Verification items for the finished model (mm, model axes). Face numbers are marked on the shaded views. Give positions to 0.01 mm unless a question says otherwise; leave off trailing zeros. Write each loop counter-clockwise with the first axis right and the second up, starting at its lowest first coordinate (ties: lowest second). Pieces come first, ordered by that corner, then holes. Notation, with made-up numbers: (-20, 72) -> (-2, 72) arc R22 cw to (-2, 79) -> close; hole circle Ø3 at (43.5, 89). An arc over 180 degrees is marked (long way). Use CSV: the item, a comma, the result in double quotes. Start each with the question number.
```python
from build123d import *

# Parameters (mm, degrees)
SKETCH1_R           = 25
BOSS_EXTRUDE1_DEPTH = 3.175
SKETCH2_W           = 4.5
SKETCH2_H           = 2.5
CUT_EXTRUDE1_DEPTH  = 0.5


with BuildPart() as part:
    # Sketch1 → Boss-Extrude1 (new body)
    with BuildSketch(Plane(origin=(0, 0, 0), x_dir=(1, 0, 0), z_dir=(0, 1, 0))):
        Circle(SKETCH1_R)
    extrude(amount=BOSS_EXTRUDE1_DEPTH)

    # Sketch2 → Cut-Extrude1 (cut)
    with BuildSketch(Plane(origin=(0, 3.175, 0), x_dir=(1, 0, 0), z_dir=(0, 1, 0))):
        with BuildLine():
            Line((17.25, 0.25), (17.25, -5.855662433))
            Line((17.25, -5.855662433), (18.049038106, -6.316987298))
            Line((18.049038106, -6.316987298), (18.049038106, -5.25))
            Line((18.049038106, -5.25), (18.049038106, -4.816987298))
            Line((18.049038106, -4.816987298), (18.549038106, -4.816987298))
            Line((18.549038106, -4.816987298), (18.549038106, -5.25))
            Line((18.549038106, -5.25), (18.549038106, -6.5))
            Line((18.549038106, -6.5), (21.299038106, -6.5))
            Line((21.299038106, -6.5), (21.299038106, -7))
            Line((21.299038106, -7), (18.549038106, -7))
            Line((18.549038106, -7), (18.549038106, -8.25))
            Line((18.549038106, -8.25), (18.549038106, -8.683012702))
            Line((18.549038106, -8.683012702), (18.049038106, -8.683012702))
            Line((18.049038106, -8.683012702), (18.049038106, -8.25))
            Line((18.049038106, -8.25), (18.049038106, -7.183012702))
            Line((18.049038106, -7.183012702), (15.450961894, -8.683012702))
            Line((15.450961894, -8.683012702), (15.450961894, -7))
            Line((15.450961894, -7), (12.700961894, -7))
            Line((12.700961894, -7), (12.700961894, -6.5))
            Line((12.700961894, -6.5), (15.450961894, -6.5))
            Line((15.450961894, -6.5), (15.450961894, -4.816987298))
            Line((15.450961894, -4.816987298), (16.75, -5.566987298))
            Line((16.75, -5.566987298), (16.75, -0.25))
            Line((16.75, -0.25), (0.25, -0.25))
            Line((0.25, -0.25), (0.25, -24.998749969))
            ThreePointArc((0.25, -24.998749969), (0, -25), (-0.25, -24.998749969))
            Line((-0.25, -24.998749969), (-0.25, -0.25))
            Line((-0.25, -0.25), (-2.75, -0.25))
            Line((-2.75, -0.25), (-2.75, -3.25))
            Line((-2.75, -3.25), (-8.25, -3.25))
            Line((-8.25, -3.25), (-8.25, 0.25))
            Line((-8.25, 0.25), (-5.589373118, 0.25))
            Line((-5.589373118, 0.25), (-0.853083665, 4.132571689))
            Line((-0.853083665, 4.132571689), (-0.751596944, 4.215765395))
            Line((-0.751596944, 4.215765395), (-0.625482869, 4.179488852))
            Line((-0.625482869, 4.179488852), (13.035241579, 0.25))
            Line((13.035241579, 0.25), (17.25, 0.25))
        make_face()
        Polygon((-4.800684576, 0.25), (-0.297938398, 0.25), (-0.866588339, 3.47497407), align=None, mode=Mode.SUBTRACT)
        Polygon((0.209774908, 0.25), (-0.378852437, 3.588271558), (11.226526686, 0.25), align=None, mode=Mode.SUBTRACT)
        with Locations((-5.5, -1.5)):
            Rectangle(SKETCH2_W, SKETCH2_H, mode=Mode.SUBTRACT)
    extrude(amount=-CUT_EXTRUDE1_DEPTH, mode=Mode.SUBTRACT)


solid = part.part
```
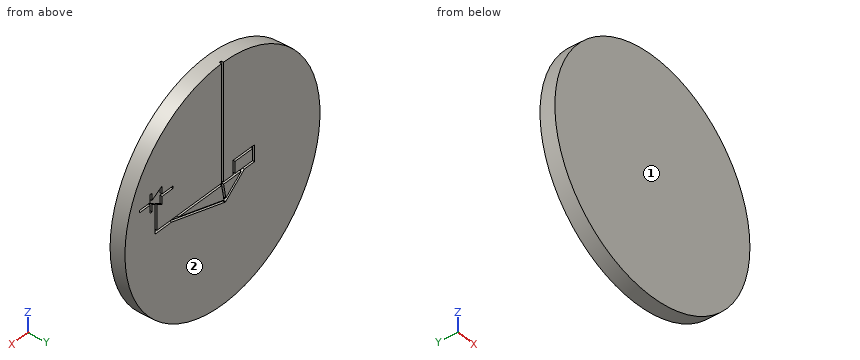
(1) Section check B-B on x = -4. Record the cut outline in (y, z) (3 decimals).
(2) Thickness scan on line 1 (Z direction, x = 16.5, y = 2.85); line 2 (Z direction, x = -0.5, y = 0.8) (3 decimals); line 3 (Z direction, x = -16.5, y = 2.7). Record the ranges inside material, lowest first. Write a range as from..to.
(3) Section check D-D on z = 11.5. Record the cut outline in (x, y) (3 decimals).
(4) Draft check along Y on the marked faces 1 and 2. Enter one of: released by +Y, released by -Y, zero draft, split by the parting line, or undercut.
(5) Section check C-C on y = 1.25. Record the cut outline in (x, z), then the cut area to 3 significant figures.
(6) Section check A-A on z = 18. Record the cut outline in (x, y) (3 decimals), then the cut area to 3 significant figures.
(7) Go/stop test with flat-tipped pins: pin 1 (0.6 mm diameter, centred on x = -5, y = 3, fed in from -Z); pin 2 (0.6 mm diameter, centred on x = -2, y = 3, fed in from -Z); pin 3 (3 mm diameter, centred on x = 4.5, z = 13.5, fed in from -Y); pin 4 (0.6 mm diameter, centred on y = 3, z = 1.5, fed in from -X). Record where each tip stops, or that it passes through.
Data:
1,outline,"(0, -24.678) -> (3.175, -24.678) -> (3.175, -1.553) -> (2.675, -1.553) -> (2.675, -0.906) -> (3.175, -0.906) -> (3.175, -0.25) -> (2.675, -0.25) -> (2.675, 0.25) -> (3.175, 0.25) -> (3.175, 2.75) -> (2.675, 2.75) -> (2.675, 3.25) -> (3.175, 3.25) -> (3.175, 24.678) -> (0, 24.678) -> close"
2,line 1,"z = -18.78..-0.25, 0.25..5.42, 8.08..18.78"
2,line 2,"z = -24.995..24.995"
2,line 3,"z = -18.78..18.78"
3,outline,"(-22.198, 0) -> (22.198, 0) -> (22.198, 3.175) -> (0.25, 3.175) -> (0.25, 2.675) -> (-0.25, 2.675) -> (-0.25, 3.175) -> (-22.198, 3.175) -> close"
4,face 1,"released by -Y"
4,face 2,"released by +Y"
5,outline,"circle Ø50 at (0, 0)"
5,area,"1,960 mm2"
6,outline,"(-17.349, 0) -> (17.349, 0) -> (17.349, 3.175) -> (0.25, 3.175) -> (0.25, 2.675) -> (-0.25, 2.675) -> (-0.25, 3.175) -> (-17.349, 3.175) -> close"
6,area,"110 mm2"
7,pin 1,"stops at z = -24.55"
7,pin 2,"stops at z = -24.94"
7,pin 3,"stops at y = 0"
7,pin 4,"stops at x = -24.97"
